from build123d import *

# Parameters (mm, degrees)
F1_DEPTH = 5.7912
F3_DEPTH = 3.2512


with BuildPart() as f1:
    # F0 (on Right) → F1 (new body)
    with BuildSketch(Plane.YZ):
        with BuildLine():
            Line((20.32, 0.3259240077), (3.0216997567, 13.1259928519))
            ThreePointArc((3.0216997567, 13.1259928519), (1.5908721369, 13.8668715611), (0, 14.1224))
            ThreePointArc((0, 14.1224), (-1.5908721369, 13.8668715611), (-3.0216997567, 13.1259928519))
            Line((-3.0216997567, 13.1259928519), (-20.32, 0.3259240077))
            Line((-20.32, 0.3259240077), (-20.32, -13.7964759923))
            Line((-20.32, -13.7964759923), (-3.0216997567, -0.9964071481))
            ThreePointArc((-3.0216997567, -0.9964071481), (-1.5908721369, -0.2555284389), (0, 0))
            ThreePointArc((0, 0), (1.5908721369, -0.2555284389), (3.0216997567, -0.9964071481))
            Line((3.0216997567, -0.9964071481), (20.32, -13.7964759923))
            Line((20.32, -13.7964759923), (20.32, 0.3259240077))
        make_face()
    extrude(amount=F1_DEPTH)

    # F2 (on face) → F3 (cut)
    with BuildSketch(Plane.YZ.offset(5.7912)):
        Polygon((19.2532, -13.0070855174), (20.32, -13.7964759923), (20.32, 0.3259240077), (19.2532, 1.1153144826), align=None)
        Polygon((-19.2532, -13.0070855174), (-19.2532, 1.1153144826), (-20.32, 0.3259240077), (-20.32, -13.7964759923), align=None)
    extrude(amount=-F3_DEPTH, mode=Mode.SUBTRACT)


solid = f1.part
Can you work these out from the model? Positions are in its coordinate system, mm. A direction names the side the tool comes from. Round coordinates to 2 decimals unless told otherwise and drop trailing zeros. Write each loop counter-clockwise with the first axis right and the second up, starting at its lowest first coordinate (ties: lowest second). Pieces come first, ordered by that corner, then holes. Notation, with made-up numbers: M 13.5,81 L 60.5,81 A34 ccw 60.5,114 Z; hole C 67.25,-7.75 d6. An arc over 180 degrees is marked long. Use a Markdown table: item, result.
Item 1: If I drill on line 1 along Y through (x, z) = (2.9, -9.75); line 2 along Y through (x, z) = (2.15, -6.25); line 3 along Y through (x, z) = (3.55, 1), over which ranges is the centre line in solid material (lowest first)? Write a range as [from, to].
Found:
| item | result |
|---|---|
| line 1 | y = [-19.25, -14.85], [14.85, 19.25] |
| line 2 | y = [-20.32, -10.12], [10.12, 20.32] |
| line 3 | y = [-19.25, 19.25] |
Item 2: I want a section at A-A (x = 1.25). List the corners of the cut face in (y, z) for me, and give its area (3 significant figures).
Found:
| item | result |
|---|---|
| outline | M -20.32,-13.8 L -3.02,-1 A5.08 cw 3.02,-1 L 20.32,-13.8 L 20.32,0.33 L 3.02,13.13 A5.08 ccw -3.02,13.13 L -20.32,0.33 Z |
| area | 574 mm2 |
Item 3: We'd pull the mould along Y, two halves only. Please class faces 1 (the face through (2.855, -11.792, -7.486)), 2 (the face through (0, -0.3, 0.4)), 3 (the face through (1, 20.32, -7)), 4 (the face through (2.855, -11.55, 6.816)): released by +Y, released by -Y, zero draft, split by the parting line, or undercut.
Found:
| item | result |
|---|---|
| face 1 | undercut |
| face 2 | zero draft |
| face 3 | released by +Y |
| face 4 | released by -Y |
Item 4: I want a section at B-B (z = 9.75). List the corners of the cut face in (x, y) for me.
Found:
| item | result |
|---|---|
| outline | M 0,-7.58 L 5.79,-7.58 L 5.79,7.58 L 0,7.58 Z |
Item 5: I want a section at C-C (x = 4). List the corners of the cut face in (y, z) for me, and give its area (3 significant figures).
Found:
| item | result |
|---|---|
| outline | M -19.25,-13.01 L -3.02,-1 A5.08 cw 3.02,-1 L 19.25,-13.01 L 19.25,1.12 L 3.02,13.13 A5.08 ccw -3.02,13.13 L -19.25,1.12 Z |
| area | 544 mm2 |
Item 6: I want a section at D-D (y = -13.5). List the corners of the cut face in (x, z) for me, and give its area (3 significant figures).
Found:
| item | result |
|---|---|
| outline | M 0,-8.75 L 5.79,-8.75 L 5.79,5.37 L 0,5.37 Z |
| area | 81.8 mm2 |
Item 7: Which directions (+Z, -Z, +X, -X, +Y, -Y) give clear straight access to the entire face, cutting with the end or side of a thin tool? Please do faces 5 (the face through (4, 19.253, -6)), 6 (the face through (2.855, 11.55, -7.307)), 7 (the face through (4, -19.253, -6)).
Found:
| item | result |
|---|---|
| face 5 | +Z, -Z, +X, +Y |
| face 6 | -Z, +X, -X |
| face 7 | +Z, -Z, +X, -Y |
Item 8: For pin 1 Ø1.2 at (y, z) = (20, -7.5) entering from +X; pin 2 Ø1 at (x, z) = (3, 4.5) entering from -Y, each with a flat end and sliding along its axis, tell me the tip position at first contact or that it passes through.
Found:
| item | result |
|---|---|
| pin 1 | stops at x = 2.54 |
| pin 2 | stops at y = -15.35 |
